Autodesk Inventor part; units mm, degrees
ref_plane "YZ Plane" through (0, 0, 0) normal (1, 0, 0) x (0, 1, 0)
ref_plane "XZ Plane" through (0, 0, 0) normal (0, 1, 0) x (-1, 0, 0)
ref_plane "XY Plane" through (0, 0, 0) normal (0, 0, 1) x (1, 0, 0)
sketch "Sketch1" plane through (0, 0, 0) normal (0, 1, 0) x (-1, 0, 0)
  line L0 (0, 0) -> (-94, 0)
  line L1 (-94, 0) -> (-94, -87)
  line L2 (-94, -87) -> (0, -87)
  line L3 (0, -87) -> (0, 0)
  dimension "d0" = 94
  dimension "d1" = 87
extrude "Extrusion1" add sketch "Sketch1" along normal blind 2
sketch "Sketch2" plane through (0, 0, 0) normal (0, 0, 1) x (1, 0, 0)
  line L0 (94, 2) -> (0, 2)
  line L1 (-0.0001, 2) -> (94, 2)
  line L2 (94, 2) -> (99, 7)
  line L3 (94, 2) -> (101.071, 2) construction
  line L4 (94, 0) -> (99, 5)
  line L5 (99, 5) -> (114, 5)
  line L6 (114, 5) -> (114, 7)
  line L7 (114, 7) -> (99, 7)
  line L8 (94, 0) -> (94, 2)
  line L9 (94, 0) -> (94, 2)
  point P0 (0, 0)
  dimension "d4" = 7.071
  dimension "d5" = 45
  dimension "d6" = 7.071
  dimension "d7" = 15
  dimension "d8" = 2
extrude "Extrusion2" add sketch "Sketch2" against normal blind 87
sketch "Sketch3" plane through (99, 7, 0) normal (0, 1, 0) x (1, 0, 0)
  line L0 (15, 0) -> (0, 0)
  line L1 (15, 0) -> (20, 5)
  line L2 (15, 0) -> (22.071, 0) construction
  line L3 (20, 5) -> (20, 82)
  line L4 (0, 87) -> (15, 87)
  line L5 (20, 82) -> (15, 87)
  line L6 (15, 0) -> (15, 87)
  point P0 (-99, 0)
  dimension "d11" = 7.071
  dimension "d12" = 45
  dimension "d13" = 77
extrude "Extrusion3" add sketch "Sketch3" against normal blind 2
equation "\"BendRadius\" = Thickness"
equation "\"BendReliefWidth\" = Thickness"
equation "\"BendReliefDepth\" = 0.5 * Thickness"
equation "\"CornerReliefSize\" = 4 * Thickness"
equation "\"MinimumRemnant\" = 2 * Thickness"
equation "\"TransitionRadius\" = BendRadius"
equation "\"JacobiRadiusSize\" = BendRadius"
equation "\"GapSize\" = Thickness"
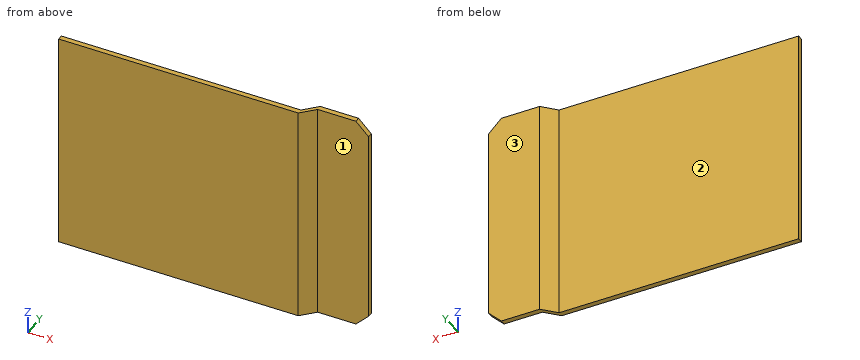
Read the model definition and answer for the solid it produces. Units are mm, in the model's axes. Face numbers are marked on the shaded views. A direction names the side the tool comes from. Round coordinates to 2 decimals unless told otherwise and drop trailing zeros. Order: outer loops, then holes, each group sorted by start corner. A loop starts at its lowest first (then second) coordinate and runs counter-clockwise, first axis right, second up.
1) Straight lines are drawn through the part: L1, parallel to Y at x = 112, z = -7.5; L2, parallel to Y at x = 73, z = -4.5; L3, parallel to X at y = 3.5, z = -43. For each, find the intervals that lie inside material, in ascending order.
2) The part is cut by section A-A on z = -77. Write down the section's boundary in (x, y).
3) The part is cut by section B-B on x = 38.5. Write down the section's boundary in (y, z).
4) The part is cut by section C-C on y = 3.75. Write down the section's boundary in (x, z), plus the area to 3 significant figures.
5) For the marked faces 1, 2 and 3, determine the directions among +Z, -Z, +X, -X, +Y, -Y from which every point of the face is accessible in a straight line to the end or side of a thin tool.
6) A flat-ended cylindrical pin translates along its axis: pin 1 (6 mm diameter, centred on x = 108, z = -52.5, fed in from -Y). Find the tip coordinate at first contact, or state that the pin passes through.
Resolved:
1. L1: y = 5 to 7
1. L2: y = 0 to 2
1. L3: x = 95.5 to 97.5
2. outline: (0, 0) - (94, 0) - (99, 5) - (119, 5) - (119, 7) - (99, 7) - (94, 2) - (0, 2) - close
3. outline: (0, -87) - (2, -87) - (2, 0) - (0, 0) - close
4. outline: (95.75, -87) - (97.75, -87) - (97.75, 0) - (95.75, 0) - close
4. area: 174 mm2
5. face 1: +Z, -Z, +X, -Y
5. face 2: +Z, -Z, -X, +Y
5. face 3: +Z, -Z, +X, -X, +Y
6. pin 1: stops at y = 5
